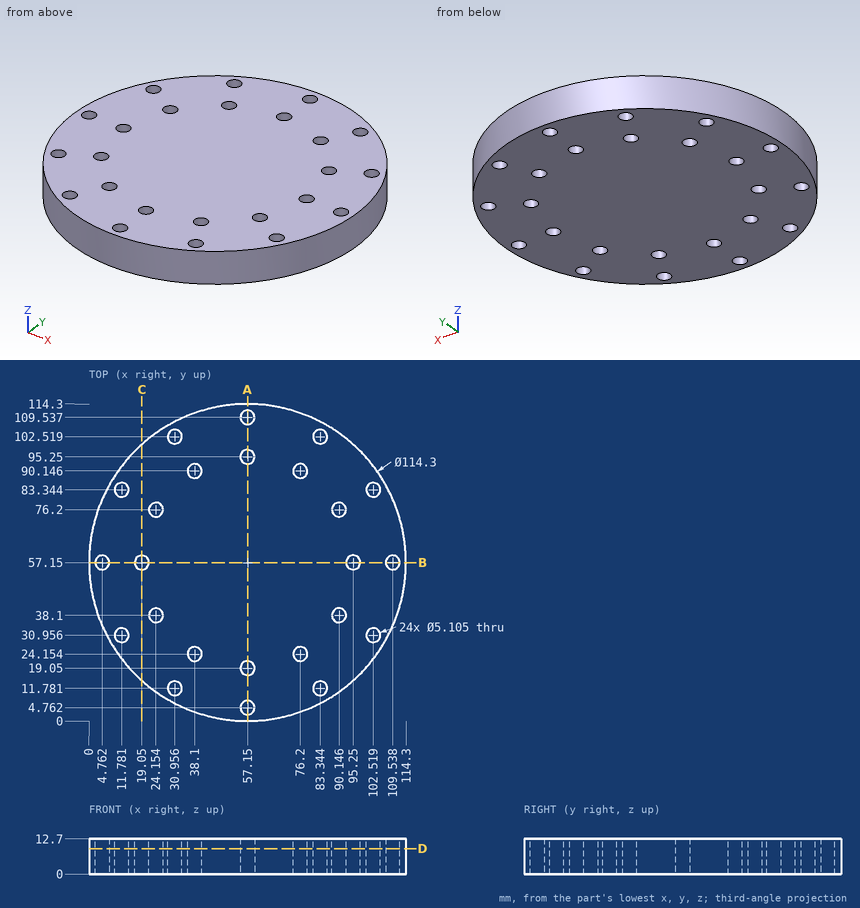
Can you work these out from the drawing? Everything is in mm from the part's minimum corner. Round coordinates to 2 decimals unless told otherwise and drop trailing zeros. Order: outer loops, then holes, each group sorted by start corner. A loop starts at its lowest first (then second) coordinate and runs counter-clockwise, first axis right, second up. Notation, with made-up numbers: (67, 70.5) -> (77, 70.5) arc R6 cw to (77, 80.5) -> close; hole circle Ø2 at (67.25, 78). An arc over 180 degrees is marked (long way). Return JSON: item names as keys, results as strings. Group by question number.
1. If we section it at A-A, the plane x = 57.15: Write out the boundary of the cut face in (y, z) (1 decimal).
2. If we section it at D-D, the plane z = 9.25: Count the separate pieces of the cut face and the enclosed holes in it, then the cut area to 3 significant figures.
3. I need wall thicknesses on line 1 (Y direction, x = 39.5, z = 4.5) (1 decimal); line 2 (X direction, y = 76, z = 1.5); line 3 (X direction, y = 31.5, z = 7) (1 decimal). Which ranges of each line are inside material? Lowest first, please. Write a range as [from, to].
4. If we section it at C-C, the plane x = 19.05: Write out the boundary of the cut face in (y, z), then the cut area to 3 significant figures.
5. Will these pins go through, and if not, where does the flat tip stop? pin 1 (6 mm diameter, centred on y = 95, z = 10.5, fed in from +X) (1 decimal); pin 2 (3 mm diameter, centred on x = 90.5, z = 1.5, fed in from -Y); pin 3 (3 mm diameter, centred on x = 98.5, z = 10.5, fed in from -Y) (1 decimal).
Output values:
{
 "1": {"outline": "(0, 0) -> (2.2, 0) -> (2.2, 12.7) -> (0, 12.7) -> close; (7.3, 0) -> (16.5, 0) -> (16.5, 12.7) -> (7.3, 12.7) -> close; (21.6, 0) -> (92.7, 0) -> (92.7, 12.7) -> (21.6, 12.7) -> close; (97.8, 0) -> (107, 0) -> (107, 12.7) -> (97.8, 12.7) -> close; (112.1, 0) -> (114.3, 0) -> (114.3, 12.7) -> (112.1, 12.7) -> close"},
 "2": {"separate pieces": "1", "enclosed holes": "24", "area": "9,770 mm²"},
 "3": {"line 1": "[2.8, 22], [26.3, 88], [92.3, 111.5]", "line 2": "[3.2, 21.61], [26.7, 87.6], [92.69, 111.1]", "line 3": "[6.1, 9.3], [14.3, 100], [105, 108.2]"},
 "4": {"outline": "(14.55, 0) -> (54.6, 0) -> (54.6, 12.7) -> (14.55, 12.7) -> close; (59.7, 0) -> (99.75, 0) -> (99.75, 12.7) -> (59.7, 12.7) -> close", "area": "1,020 mm²"},
 "5": {"pin 1": "x = 102.4", "pin 2": "y = 9.7", "pin 3": "y = 16.2"}
}
